Part model, mm, in its own coordinate system. A direction names the side the tool comes from. Coordinates: 2 decimals unless noted, no trailing zeros. Loops run counter-clockwise (first coordinate to the right, second up) from the corner with the lowest first, then second, coordinate; pieces in that order, holes last. Notation, with made-up numbers: (72.5, 22) -> (130.5, 22) arc R18 cw to (130.5, 33) -> close; hole circle Ø8 at (75, 10.5). An arc over 180 degrees is marked (long way). Use one line per item in the form item = value. Start each with the question number.
(1) Drill centre lines: L1, parallel to X at y = 24, z = -0.25; L2, parallel to Y at x = -151.5, z = 5; L3, parallel to Z at x = 114.5, y = 49.5. Where is each one in solid material? Low to high. Write a range as [from, to].
(2) Band-saw the part on C-C on x = -7.5. Give the cut face in (y, z).
(3) Pin check, flat tips, straight feed: P1, Ø1.6, axis at x = 188.5, z = -0.5, coming from the -Y side; P2, Ø0.9, axis at y = -58, z = 1, coming from the +X side; P3, Ø10, axis at x = 74.5, y = -5, coming from the +Z side; P4, Ø3, axis at y = -3, z = 3, coming from the -X side. Stop position of each tip, or through.
(4) Band-saw the part on A-A on x = 190. Give the cut face in (y, z), then the cut area to 4 significant figures.
(5) Band-saw the part on B-B on y = 32. Give the cut face in (x, z), then the cut area to 3 significant figures.
(6) 3-axis set-ups, long thin cutter, end or side, ignore diameter. For faces 1 (the cylindrical face through (-169.15, -59.24, 9.49)), 2 (the flat face through (-2, -58.5, 7)): which of +Z, -Z, +X, -X, +Y, -Y reach the whole face in a straight line?
```python
from build123d import *

# Parameters (mm, degrees)
SKETCH_1_W                       = 410
SKETCH_1_H                       = 120
SM_BASE_FLANGE_1_DEPTH           = 1.5
SM_EDGE_FLANGE_1_STRIP_W         = 9.2
SM_EDGE_FLANGE_1_STRIP_H         = 1.5
SM_EDGE_FLANGE_1_STRIP_CUT_DEPTH = 410
SM_EDGE_FLANGE_1_DEPTH           = 410
SKETCH_8_W                       = 33
SKETCH_8_H                       = 14
CUT_EXTRUDE_1_DEPTH              = 3.1
FILLET_2_R                       = 10
CUT_EXTRUDE_3_DEPTH              = 10


# Sheet-metal steps are written as plain solids
with BuildPart() as part:
    # Sketch 1 → Базовая кромка1 (new body)
    with BuildSketch(Plane.XY):
        Rectangle(SKETCH_1_W, SKETCH_1_H)
    extrude(amount=-SM_BASE_FLANGE_1_DEPTH)

    # Ребро-кромка1 strip (across the edge) → Ребро-кромка1 strip cut (cut)
    with BuildSketch(Plane(origin=(-205, -60, 0), x_dir=(0, 1, 0), z_dir=(1, 0, 0))):
        with Locations((-1.5, -0.75)):
            Rectangle(SM_EDGE_FLANGE_1_STRIP_W, SM_EDGE_FLANGE_1_STRIP_H)
    extrude(amount=SM_EDGE_FLANGE_1_STRIP_CUT_DEPTH, mode=Mode.SUBTRACT)

    # Ребро-кромка1 section (across the edge) → Ребро-кромка1 (add)
    with BuildSketch(Plane(origin=(-205, -60, 0), x_dir=(0, 1, 0), z_dir=(1, 0, 0))):
        with BuildLine():
            Line((0, 1.6), (0, 12.5))
            Line((0, 12.5), (1.5, 12.5))
            Line((1.5, 12.5), (1.5, 1.6))
            ThreePointArc((1.5, 1.6), (1.96862915, 0.46862915), (3.1, 0))
            Line((3.1, 0), (3.1, -1.5))
            ThreePointArc((3.1, -1.5), (0.907968978, -0.592031022), (0, 1.6))
        make_face()
    extrude(amount=SM_EDGE_FLANGE_1_DEPTH)

    # Эскиз8 → Вырез-Вытянуть1 (cut)
    with BuildSketch(Plane(origin=(0, -60, 0), x_dir=(1, 0, 0), z_dir=(0, 1, 0))):
        with Locations((-188.5, -5.5)):
            Rectangle(SKETCH_8_W, SKETCH_8_H)
        with Locations((188.5, -5.5)):
            Rectangle(SKETCH_8_W, SKETCH_8_H)
    extrude(amount=CUT_EXTRUDE_1_DEPTH, mode=Mode.SUBTRACT)

    # Скругление2
    fillet_2_edges = [part.edges().sort_by_distance(p)[0] for p in [
        (-205, -56.9, -0.75),
        (205, -56.9, -0.75),
        (-172, -59.25, 12.5),
        (-205, 60, -0.75),
        (205, 60, -0.75),
        (172, -59.25, 12.5),
    ]]
    fillet(fillet_2_edges, radius=FILLET_2_R)

    # Эскиз13 → Вырез-Вытянуть3 (cut)
    with BuildSketch(Plane.XY):
        with BuildLine():
            Line((-186.5, 40), (-186.5, -40))
            ThreePointArc((-186.5, -40), (-190, -43.5), (-193.5, -40))
            Line((-193.5, -40), (-193.5, 40))
            ThreePointArc((-193.5, 40), (-190, 43.5), (-186.5, 40))
        make_face()
        with BuildLine():
            Line((186.5, 40), (186.5, -40))
            ThreePointArc((186.5, -40), (190, -43.5), (193.5, -40))
            Line((193.5, -40), (193.5, 40))
            ThreePointArc((193.5, 40), (190, 43.5), (186.5, 40))
        make_face()
    extrude(amount=-CUT_EXTRUDE_3_DEPTH, mode=Mode.SUBTRACT)


solid = part.part
```
A:
q1.L1 = [-205, -193.5], [-186.5, 186.5], [193.5, 205]
q1.L2 = [-60, -58.5]
q1.L3 = [-1.5, 0]
q2.outline = (-60, 1.6) arc R3.1 ccw to (-56.9, -1.5) -> (60, -1.5) -> (60, 0) -> (-56.9, 0) arc R1.6 cw to (-58.5, 1.6) -> (-58.5, 12.5) -> (-60, 12.5) -> close
q3.P1 = -56.9
q3.P2 = 172
q3.P3 = 0
q3.P4 = through
q4.outline = (-56.9, -1.5) -> (-43.5, -1.5) -> (-43.5, 0) -> (-56.9, 0) -> close; (43.5, -1.5) -> (60, -1.5) -> (60, 0) -> (43.5, 0) -> close
q4.area = 44.85 mm²
q5.outline = (-205, -1.5) -> (-193.5, -1.5) -> (-193.5, 0) -> (-205, 0) -> close; (-186.5, -1.5) -> (186.5, -1.5) -> (186.5, 0) -> (-186.5, 0) -> close; (193.5, -1.5) -> (205, -1.5) -> (205, 0) -> (193.5, 0) -> close
q5.area = 594 mm²
q6.face_1 = +Z, -X, +Y, -Y
q6.face_2 = +Z, +X, -X, +Y
